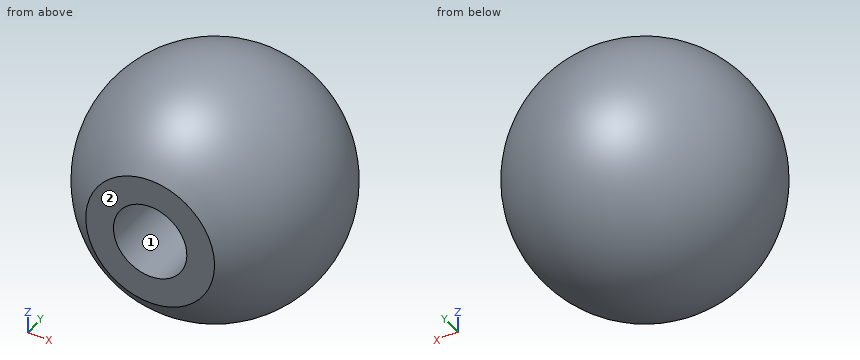
from build123d import *

# Parameters (mm, degrees)
SKETCH_2_W          = 12
SKETCH_2_H          = 3
CUT_EXTRUDE_1_DEPTH = 6
SKETCH_3_R          = 3
CUT_EXTRUDE_2_DEPTH = 15


with BuildPart() as part:
    # Эскиз1 → Revolve 273 (revolve)
    with BuildSketch(Plane.XY):
        with BuildLine():
            Line((0, 10), (0, 0))
            Line((0, 0), (0, -10))
            ThreePointArc((0, -10), (10, 0), (0, 10))
        make_face()
    revolve(axis=Axis((0, 10, 0), (0, -1, 0)))

    # Эскиз2 → Вырез-Вытянуть1 (cut, symmetric)
    with BuildSketch(Plane.XY):
        with Locations((0, -10)):
            Rectangle(SKETCH_2_W, SKETCH_2_H)
    extrude(amount=CUT_EXTRUDE_1_DEPTH, both=True, mode=Mode.SUBTRACT)

    # Эскиз3 → Вырез-Вытянуть2 (cut)
    with BuildSketch(Plane.XZ.offset(8.5)):
        with Locations(Location((0, 0, 0), (0, 0, 270))):
            Circle(SKETCH_3_R)
    extrude(amount=-CUT_EXTRUDE_2_DEPTH, mode=Mode.SUBTRACT)


solid = part.part
Design review of the part built by this model. Coordinates are the model's own, in mm. Face numbers are marked on the shaded views. Round coordinates to 2 decimals unless told otherwise and drop trailing zeros. Write each loop counter-clockwise with the first axis right and the second up, starting at its lowest first coordinate (ties: lowest second). Pieces come first, ordered by that corner, then holes.
Item 1: Consider section C-C on y = 0.5. Give the boundary of the cut face in (x, z), and give its area (3 significant figures).
Item 2: Consider section A-A on z = 0. Give the boundary of the cut face in (x, y), and give its area (3 significant figures).
Item 3: For pin 1 Ø3 at (x, z) = (4.5, 7.5) entering from +Y; pin 2 Ø10 at (y, z) = (-0.5, -6) entering from -X; pin 3 Ø10 at (x, y) = (0.5, 5.5) entering from +Z, all flat-tipped, find the tip position at first contact; note any pin that passes through.
Item 4: Consider section B-B on x = 0. Give the boundary of the cut face in (y, z).
Item 5: Consider section D-D on y = -4.25. Give the boundary of the cut face in (x, z).
Item 6: Draft analysis for pull direction X (two halves, no side actions). For the marked faces 1 and 2, state which applies: released by +X, released by -X, zero draft, split by the parting line, or undercut.
Item 7: Wall thickness on L1, parallel to X at y = 0, z = 0; L2, parallel to X at y = -4.75, z = 0; L3, parallel to Z at x = 2, y = -7.25: over which ranges is each line inside the solid? List them lowest first.
Check values:
1. outline: circle Ø19.97 at (0, 0); hole circle Ø6 at (0, 0)
1. area: 285 mm2
2. outline: (-5.27, -8.5) - (-3, -8.5) - (-3, 6.5) - (3, 6.5) - (3, -8.5) - (5.27, -8.5) arc R10 ccw (long way) to start
2. area: 213 mm2
3. pin 1: stops at y = 6.89
3. pin 2: stops at x = -9.95
3. pin 3: stops at z = 9.99
4. outline: (-8.5, -5.27) arc R10 ccw (long way) to (-8.5, 5.27) - (-8.5, 3) - (6.5, 3) - (6.5, -3) - (-8.5, -3) - close
5. outline: circle Ø18.1 at (0, 0); hole circle Ø6 at (0, 0)
6. face 1: undercut
6. face 2: zero draft
7. L1: x = -10 to -3, 3 to 10
7. L2: x = -8.8 to -3, 3 to 8.8
7. L3: z = -6.59 to -2.24, 2.24 to 6.59
